```python
from build123d import *

# Parameters (mm, degrees)
F1_DEPTH  = 3.2004
F2_T      = -1.524
F3_R      = 2.4384
F4_DEPTH  = 1.7526
F5_R      = 1.3
F6_DEPTH  = 1.7
F8_DEPTH  = 1.524
F9_R      = 1.5367
F10_DEPTH = 1.524
F11_R     = 0.762
F12_DEPTH = 1.524
F13_R     = 0.762
F14_DEPTH = 1.524


with BuildPart() as f1:
    # F0 (on Top) → F1 (new body)
    with BuildSketch(Plane.XY):
        Polygon((-7.8994, -7.8994), (0, -7.8994), (0, 0), (7.9248, 0), (7.9248, 7.8994), (-7.8994, 7.8994), (-7.8994, 0), align=None)
    extrude(amount=F1_DEPTH)

    # F2
    f2_openings = [f1.faces().sort_by_distance(p)[0] for p in [
        (-1.306686, 1.319386, 0),
    ]]
    offset(amount=F2_T, openings=f2_openings, kind=Kind.INTERSECTION)

    # F3 (on face) → F4 (join)
    with BuildSketch(Plane.XY.offset(3.2004)):
        with Locations((3.9624, 3.9497)):
            Circle(F3_R)
        with Locations((-3.9497, 3.9497)):
            Circle(F3_R)
        with Locations((-3.9497, -3.9497)):
            Circle(F3_R)
    extrude(amount=F4_DEPTH)

    # F5 (on face) → F6 (cut)
    with BuildSketch(Plane(origin=(0, 0, 0), x_dir=(1, 0, 0), z_dir=(0, 0, -1))):
        with Locations((-3.9497, 3.9497)):
            Circle(F5_R)
        with Locations((-3.9497, -3.9497)):
            Circle(F5_R)
        with Locations((3.9624, -3.9497)):
            Circle(F5_R)
    extrude(amount=-F6_DEPTH, mode=Mode.SUBTRACT)

    # F7 (on face) → F8 (join)
    with BuildSketch(Plane(origin=(0, 0, 1.6764), x_dir=(1, 0, 0), z_dir=(0, 0, -1))):
        Polygon((-0.7157769491, -1.524), (-1.524, -0.7157769491), (-2.5297886856, -1.7215656347), (-1.7215656347, -2.5297886856), align=None)
    extrude(amount=F8_DEPTH)

    # F9 (on face) → F10 (join)
    with BuildSketch(Plane(origin=(0, 0, 1.6764), x_dir=(1, 0, 0), z_dir=(0, 0, -1))):
        with Locations((-3.9497, 0)):
            Circle(F9_R)
        with Locations((0, -3.9497)):
            Circle(F9_R)
    extrude(amount=F10_DEPTH)

    # F11 (on face) → F12 (cut)
    with BuildSketch(Plane(origin=(0, 0, 0.1524), x_dir=(1, 0, 0), z_dir=(0, 0, -1))):
        with Locations((-3.9497, 0)):
            Circle(F11_R)
    extrude(amount=-F12_DEPTH, mode=Mode.SUBTRACT)

    # F13 (on face) → F14 (cut)
    with BuildSketch(Plane(origin=(0, 0, 0.1524), x_dir=(1, 0, 0), z_dir=(0, 0, -1))):
        with Locations((0, -3.9497)):
            Circle(F13_R)
    extrude(amount=-F14_DEPTH, mode=Mode.SUBTRACT)


solid = f1.part
```
Geometry: final body of the model. Coordinates: model frame, mm. A direction names the side the tool comes from. Coordinates: 2 decimals unless noted, no trailing zeros. Loops run counter-clockwise (first coordinate to the right, second up) from the corner with the lowest first, then second, coordinate; pieces in that order, holes last. Notation, with made-up numbers: (14.25, 36.5) -> (71.25, 36.5) arc R29 cw to (71.25, 57.5) -> close; hole circle Ø11 at (-26, 61.5). An arc over 180 degrees is marked (long way). Use a Markdown table: item, result. Add a question column.
(1) Section query A-A, the plane z = 2.65. Return loops of the section in (x, y).
(2) Line query: line 1 along X through (y, z) = (4, 0.45); line 2 along X through (y, z) = (-1, 0.45); line 3 along X through (y, z) = (-2.75, 1.05). Output: solid intervals per line, ascending.
(3) Section query C-C, the plane z = 3.7. Return loops of the section in (x, y), plus the area to 3 significant figures.
(4) Access query for faces 1 (the flat face through (7.925, 4, 2)), 2 (the flat face through (-4, 4, 1.7)), 3 (the cylindrical face through (-5.747, -2.302, 4.064)), 4 (the flat face through (4, 0, 2)), 5 (the flat face through (-7.899, 0, 2)). Directions: +Z, -Z, +X, -X, +Y, -Y. A direction counts if a zero-diameter tool reaches every point of the face in a straight line with its end or side. Return the directions, or none.
(5) Section query B-B, the plane x = 1.25. Return loops of the section in (y, z), plus the area to 3 significant figures.
(6) Mould query, pull axis Y, two halves, no side actions, for faces 6 (the cylindrical face through (5.088, 1.786, 4.064)), 7 (the flat face through (-1, 4, 0.152)), 8 (the flat face through (-4, 4, 4.953)). Classes: pulls with the +Y half, pulls with the -Y half, needs draft (parallel to the pull), parting line crosses it, or undercut.
(7) Pin query (flat end, axial travel): pin 1 Ø1.8 at (x, z) = (0.5, 0.5) entering from -Y; pin 2 Ø1 at (x, y) = (1, 5.5) entering from +Z; pin 3 Ø2.5 at (x, y) = (-0.5, 4.5) entering from -Z; pin 4 Ø1.4 at (x, y) = (0, 3.95) entering from -Z. Return the tip coordinate at first contact, or that it passes through.
Answer:
| question | item | result |
|---|---|---|
| 1 | outline | (-7.9, -7.9) -> (0, -7.9) -> (0, 0) -> (7.92, 0) -> (7.92, 7.9) -> (-7.9, 7.9) -> close |
| 2 | line 1 | x = -7.9 to -6.38, -1.54 to -0.76, 0.76 to 1.54, 6.4 to 7.92 |
| 2 | line 2 | x = -7.9 to -6.38, -5.12 to -2.78, -1.52 to 0 |
| 2 | line 3 | x = -7.9 to -6.38, -1.52 to 0 |
| 3 | outline | circle Ø4.88 at (-3.95, -3.95); circle Ø4.88 at (-3.95, 3.95); circle Ø4.88 at (3.96, 3.95) |
| 3 | area | 56.0 mm^2 |
| 4 | face 1 | +Z, -Z, +X, +Y, -Y |
| 4 | face 2 | -Z |
| 4 | face 3 | +Z |
| 4 | face 4 | +Z, -Z, +X, -Y |
| 4 | face 5 | +Z, -Z, -X, +Y, -Y |
| 5 | outline | (0, 0) -> (1.52, 0) -> (1.52, 1.68) -> (3.06, 1.68) -> (3.06, 0.15) -> (4.84, 0.15) -> (4.84, 1.68) -> (6.38, 1.68) -> (6.38, 0) -> (7.9, 0) -> (7.9, 3.2) -> (0, 3.2) -> close |
| 5 | area | 19.9 mm^2 |
| 6 | face 6 | parting line crosses it |
| 6 | face 7 | undercut |
| 6 | face 8 | needs draft |
| 7 | pin 1 | stops at y = -7.9 |
| 7 | pin 2 | stops at z = 3.2 |
| 7 | pin 3 | stops at z = 0.15 |
| 7 | pin 4 | stops at z = 1.68 |
